Could you check a few things on this model? Use its own coordinates, in mm. A direction names the side the tool comes from. Round coordinates to 2 decimals unless told otherwise and drop trailing zeros. Write each loop counter-clockwise with the first axis right and the second up, starting at its lowest first coordinate (ties: lowest second). Pieces come first, ordered by that corner, then holes. Notation, with made-up numbers: (-13.5, 34.5) - (35.5, 34.5) arc R20 cw to (35.5, 64.5) - close; hole circle Ø9 at (16.25, -14). An arc over 180 degrees is marked (long way). Put each result on its own line as item: value.
from build123d import *

# Parameters (mm, degrees)
SKETCH1_W           = 21
SKETCH1_H           = 15.7
BOSS_EXTRUDE1_DEPTH = 1.5
SKETCH2_R           = 1.5
CUT_EXTRUDE1_DEPTH  = 1.5
SKETCH3_W           = 21
SKETCH3_H           = 2.5
BOSS_EXTRUDE2_DEPTH = 8


with BuildPart() as part:
    # Sketch1 → Boss-Extrude1 (new body)
    with BuildSketch(Plane(origin=(0, 0, 0), x_dir=(1, 0, 0), z_dir=(0, 1, 0))):
        with Locations((10.5, 7.85)):
            Rectangle(SKETCH1_W, SKETCH1_H)
    extrude(amount=BOSS_EXTRUDE1_DEPTH)

    # Sketch2 → Cut-Extrude1 (cut)
    with BuildSketch(Plane(origin=(0, 1.5, 0), x_dir=(1, 0, 0), z_dir=(0, 1, 0))):
        with Locations(Location((2.5, 2.5, 0), (0, 0, 270))):
            Circle(SKETCH2_R)
        with Locations(Location((18.5, 2.5, 0), (0, 0, 270))):
            Circle(SKETCH2_R)
    extrude(amount=-CUT_EXTRUDE1_DEPTH, mode=Mode.SUBTRACT)

    # Sketch3 → Boss-Extrude2 (add)
    with BuildSketch(Plane.XZ):
        with Locations((10.5, -14.45)):
            Rectangle(SKETCH3_W, SKETCH3_H)
    extrude(amount=BOSS_EXTRUDE2_DEPTH)


solid = part.part
(1) For faces 1 (the face through (21, 0.3, -11.4)), 2 (the face through (10, 0, -7)), which set-ups out of +Z, -Z, +X, -X, +Y, -Y let a thin tool reach every point of the face, with its end or its side?
Values found:
face 1: +Z, -Z, +X, +Y, -Y
face 2: +Z, +X, -X, -Y
(2) Imagine slicing it at C-C, the plane x = 14. List the corners of the cut face in (y, z) for me.
Values found:
outline: (-8, -15.7) - (1.5, -15.7) - (1.5, 0) - (0, 0) - (0, -13.2) - (-8, -13.2) - close
(3) Imagine slicing it at B-B, the plane x = 2.5. List the corners of the cut face in (y, z) for me.
Values found:
outline: (-8, -15.7) - (1.5, -15.7) - (1.5, -4) - (0, -4) - (0, -13.2) - (-8, -13.2) - close; (0, -1) - (1.5, -1) - (1.5, 0) - (0, 0) - close
(4) Imagine slicing it at A-A, the plane z = -2.5. List the corners of the cut face in (x, y) for me, then the cut area to 3 significant figures.
Values found:
outline: (0, 0) - (1, 0) - (1, 1.5) - (0, 1.5) - close; (4, 0) - (17, 0) - (17, 1.5) - (4, 1.5) - close; (20, 0) - (21, 0) - (21, 1.5) - (20, 1.5) - close
area: 22.5 mm^2
(5) If we mould it in two halves opening along X, with no side actions, what happens to faces 3 (the face through (1.17, 0.76, -1.81)), 4 (the face through (10, -3, -15.7)), 5 (the face through (19.765, 0.76, -1.694)), 6 (the face through (0, 0.3, -11.4))? For each: pulls with the +X half, pulls with the -X half, needs draft (parallel to the pull), parting line crosses it, or undercut.
Values found:
face 3: undercut
face 4: needs draft
face 5: undercut
face 6: pulls with the -X half
(6) Imagine slicing it at D-D, the plane y = -4.75. List the corners of the cut face in (x, z) for me, then the cut area to 3 significant figures.
Values found:
outline: (0, -15.7) - (21, -15.7) - (21, -13.2) - (0, -13.2) - close
area: 52.5 mm^2
(7) I'm going to push a flat-ended pin straight in: pin 1 (2 mm diameter, centred on x = 18, z = -8.5, fed in from -Y). Where does the tip first touch, or does it pass through?
Values found:
pin 1: stops at y = 0
(8) Please list where these lines run through material, in increasing order: probe 1 along X at (y, z) = (0.5, -2.5); probe 2 along Y at (x, z) = (6.75, -7.5); probe 3 along Z at (x, y) = (12, -6). Write a range as from..to.
Values found:
probe 1: x = 0..1, 4..17, 20..21
probe 2: y = 0..1.5
probe 3: z = -15.7..-13.2
